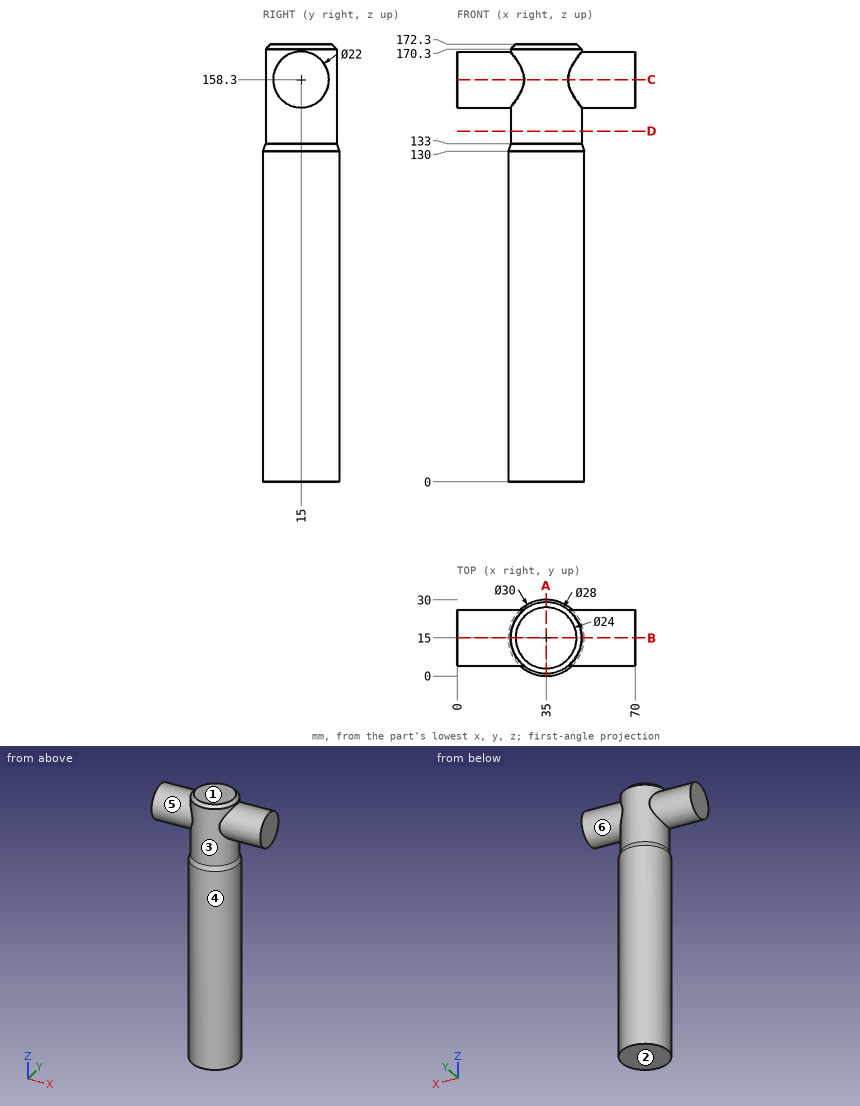
Here's the drawing with two shaded views (mm, measured from the low corner). I have some questions. A direction names the side the tool comes from. Give positions to 0.01 mm unless a question says otherwise; leave off trailing zeros. Order: outer loops, then holes, each group sorted by start corner. A loop starts at its lowest first (then second) coordinate and runs counter-clockwise, first axis right, second up. Notation, with made-up numbers: (37.25, 84.25) - (72.25, 84.25) arc R29 cw to (72.25, 121.25) - close; hole circle Ø1 at (23.25, 83). An arc over 180 degrees is marked (long way). Use a Markdown table: item, result. Add a question column.
Q1. Please list where these lines run through material, in increasing order: line 1 along Y through (x, z) = (35.5, 84.5); line 2 along X through (y, z) = (15.25, 138.5); line 3 along X through (y, z) = (15.5, 74.5).
Q2. I'm going to push flat-ended pins straight in: pin 1 (12 mm diameter, centred on y = 9, z = 80.5, fed in from -X); pin 2 (1 mm diameter, centred on x = 58, y = 6.5, fed in from +Z); pin 3 (12 mm diameter, centred on x = 19, z = 153.5, fed in from -Y). Where does each tip first touch, or does it pass through?
Q3. If we mould it in two halves opening along Z, with no side actions, what happens to the marked faces 1, 2 and 3? For each: released by +Z, released by -Z, zero draft, split by the parting line, or undercut.
Q4. If we section it at C-C on z = 158.3: Write out the boundary of the cut face in (x, y), plus the area to 3 significant figures.
Q5. If we section it at D-D on z = 138: Write out the boundary of the cut face in (x, y), plus the area to 3 significant figures.
Q6. If we section it at B-B on y = 15: Write out the boundary of the cut face in (x, z).
Q7. If we section it at A-A on x = 35: Write out the boundary of the cut face in (y, z), plus the area to 3 significant figures.
Q8. On a 3-axis mill with a long thin cutter (end or side, diameter ignored), from which of +Z, -Z, +X, -X, +Y, -Y can I reach the whole of each face in a straight line? I mean the marked faces 4, 5 and 6. Say none if no direction works.
Answers follow:
| question | item | result |
|---|---|---|
| 1 | line 1 | y = 0.01 to 29.99 |
| 1 | line 2 | x = 21 to 49 |
| 1 | line 3 | x = 20.01 to 49.99 |
| 2 | pin 1 | stops at x = 20 |
| 2 | pin 2 | stops at z = 165.85 |
| 2 | pin 3 | stops at y = 4 |
| 3 | face 1 | released by +Z |
| 3 | face 2 | released by -Z |
| 3 | face 3 | undercut |
| 4 | outline | (0, 4) - (26.34, 4) arc R14 ccw to (43.66, 4) - (70, 4) - (70, 26) - (43.66, 26) arc R14 ccw to (26.34, 26) - (0, 26) - close |
| 4 | area | 1,610 mm^2 |
| 5 | outline | circle Ø28 at (35, 15) |
| 5 | area | 616 mm^2 |
| 6 | outline | (0, 147.3) - (21, 147.3) - (21, 133) - (20, 130) - (20, 0) - (50, 0) - (50, 130) - (49, 133) - (49, 147.3) - (70, 147.3) - (70, 169.3) - (49, 169.3) - (49, 170.3) - (47, 172.3) - (23, 172.3) - (21, 170.3) - (21, 169.3) - (0, 169.3) - close |
| 7 | outline | (0, 0) - (30, 0) - (30, 130) - (29, 133) - (29, 170.3) - (27, 172.3) - (3, 172.3) - (1, 170.3) - (1, 133) - (0, 130) - close |
| 7 | area | 5,080 mm^2 |
| 8 | face 4 | -Z |
| 8 | face 5 | -X |
| 8 | face 6 | +X |
